Job drawing, mm, ordinate dimensions from the low corner. One solid piece. A direction names the side the tool comes from. Give positions to 0.01 mm unless a question says otherwise; leave off trailing zeros. Loops run counter-clockwise (first coordinate to the right, second up) from the corner with the lowest first, then second, coordinate; pieces in that order, holes last. Notation, with made-up numbers: (32.25, 59.25) - (44.25, 59.25) arc R18 ccw to (44.25, 72.25) - close; hole circle Ø2 at (34.5, 27.25). An arc over 180 degrees is marked (long way). Use a Markdown table: item, result.
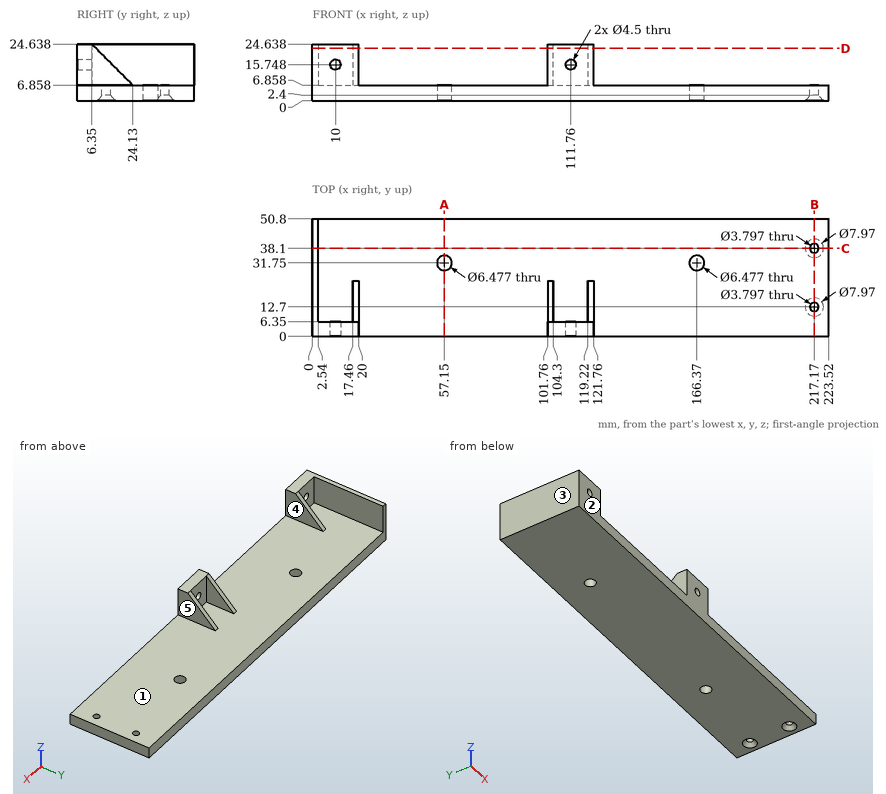
(1) Mould opens along X. For the marked faces 3, 4 and 5 say: pulls with the +X half, pulls with the -X half, needs draft (parallel to the pull), parting line crosses it, or undercut.
Computed:
| item | result |
|---|---|
| face 3 | pulls with the -X half |
| face 4 | undercut |
| face 5 | pulls with the +X half |
(2) Slice it at B-B, the plane x = 217.17. Write the cut outline in (y, z) (1 decimal), plus the area to 3 significant figures.
Computed:
| item | result |
|---|---|
| outline | (0, 0) - (8.7, 0) - (10.8, 2.4) - (10.8, 6.9) - (0, 6.9) - close; (14.6, 2.4) - (16.7, 0) - (34.1, 0) - (36.2, 2.4) - (36.2, 6.9) - (14.6, 6.9) - close; (40, 2.4) - (42.1, 0) - (50.8, 0) - (50.8, 6.9) - (40, 6.9) - close |
| area | 286 mm² |
(3) 3-axis set-ups, long thin cutter, end or side, ignore diameter. For the marked faces 1 and 2: which of +Z, -Z, +X, -X, +Y, -Y reach the whole face in a straight line?
Computed:
| item | result |
|---|---|
| face 1 | +Z, +Y |
| face 2 | +Z, -Z, +X, -X, -Y |
(4) Slice it at D-D, the plane z = 22.75. Write the cut outline in (x, y).
Computed:
| item | result |
|---|---|
| outline | (0, 0) - (20, 0) - (20, 8.24) - (17.46, 8.24) - (17.46, 6.35) - (2.54, 6.35) - (2.54, 50.8) - (0, 50.8) - close; (101.76, 0) - (121.76, 0) - (121.76, 8.24) - (119.22, 8.24) - (119.22, 6.35) - (104.3, 6.35) - (104.3, 8.24) - (101.76, 8.24) - close |
(5) Slice it at A-A, the plane x = 57.15. Write the cut outline in (y, z), plus the area to 3 significant figures.
Computed:
| item | result |
|---|---|
| outline | (0, 0) - (28.51, 0) - (28.51, 6.86) - (0, 6.86) - close; (34.99, 0) - (50.8, 0) - (50.8, 6.86) - (34.99, 6.86) - close |
| area | 304 mm² |
(6) Drill centre lines: probe 1 along Y at (x, z) = (217.17, 5.4); probe 2 along X at (y, z) = (8, 7); probe 3 along Z at (x, y) = (10, 3). Where is each one in solid material? Low to high. Write a range as [from, to].
Computed:
| item | result |
|---|---|
| probe 1 | [0, 10.8], [14.6, 36.2], [40, 50.8] |
| probe 2 | [0, 2.54], [17.46, 20], [101.76, 104.3], [119.22, 121.76] |
| probe 3 | [0, 13.5], [18, 24.64] |
(7) Pin check, flat tips, straight feed: P1, Ø7, axis at x = 111.76, z = 15.748, coming from the +Y side; P2, Ø9, axis at y = 17, z = 19.5, coming from the +X side; P3, Ø4, axis at x = 10, z = 15.748, coming from the +Y side; P4, Ø6, axis at x = 217.17, y = 38.1, coming from the -Z side. Stop position of each tip, or through.
Computed:
| item | result |
|---|---|
| P1 | y = 6.35 |
| P2 | x = 121.76 |
| P3 | through |
| P4 | z = 1.13 |
(8) Slice it at C-C, the plane y = 38.1. Write the cut outline in (x, z) (1 decimal).
Computed:
| item | result |
|---|---|
| outline | (0, 0) - (213.2, 0) - (215.3, 2.4) - (215.3, 6.9) - (2.5, 6.9) - (2.5, 24.6) - (0, 24.6) - close; (219.1, 2.4) - (221.2, 0) - (223.5, 0) - (223.5, 6.9) - (219.1, 6.9) - close |
